The listing builds one solid part. Answer for the finished solid, in the listing's coordinates (mm). A direction names the side the tool comes from. Round coordinates to 2 decimals unless told otherwise and drop trailing zeros. Order: outer loops, then holes, each group sorted by start corner. A loop starts at its lowest first (then second) coordinate and runs counter-clockwise, first axis right, second up. Notation, with made-up numbers: (68.5, 34) - (100.5, 34) arc R10 cw to (100.5, 46) - close; hole circle Ø3 at (80.25, 35). An arc over 180 degrees is marked (long way). Use CSV: the item, a comma, the result in double quotes. Start each with the question number.
Item 1: Flat-ended cylindrical pins translate along their axes: P1, Ø8, axis at x = -41.5, y = 11, coming from the -Z side; P2, Ø7.5, axis at x = 50.8, z = 50.8, coming from the -Y side; P3, Ø13.5, axis at x = 41.275, z = -41.275, coming from the +Y side. Find the tip coordinate at first contact, or state that the pin passes through.
Item 2: Find section C-C, the plane z = 1. Give the vertices of the cut face in (x, y).
Item 3: For faces 4 (the cylindrical face through (-38.167, 3.335, 38.425)), 5 (the cylindrical face through (-51.35, -2.95, -54.98)), 6 (the cylindrical face through (-61.82, 0.14, -80.63)), determine the directions among +Z, -Z, +X, -X, +Y, -Y from which every point of the face is accessible in a straight line to the end or side of a thin tool.
Item 4: Straight lines are drawn through the part: line 1 along Z through (x, y) = (54, 0.5); line 2 along Z through (x, y) = (39.5, 5); line 3 along Y through (x, z) = (34, -81.5). For each, find the intervals that lie inside material, in ascending order. Write a range as [from, to].
Item 5: Determine the mould class of faces 1 (the conical face through (50.895, 6.157, 50.074)), 2 (the flat face through (76, 10.16, 15)), 3 (the cylindrical face through (46.367, 13.917, 60.47)) for opening direction X: +X half, -X half, draft (parallel to the pull), parting line (faces both ways), or undercut.
Item 6: Find section B-B, the plane y = 15.25. Give the vertices of the cut face in (x, z) (3 decimals).
Item 7: Find section A-A, the plane x = 0. Give the vertices of the cut face in (y, z) (3 decimals), plus the area to 3 significant figures.
Item 8: Find section D-D, the plane y = 0.25. Count the separate pieces of the cut face and the enclosed holes in it, plus the area to 3 significant figures.
```python
from build123d import *

# Parameters (mm, degrees)
SKETCH1_R                   = 101.6
BOSS_EXTRUDE1_DEPTH         = 10.16
F_3_8_24_TAPPED_HOLE2_D     = 8.4328
F_3_8_24_TAPPED_HOLE2_DEPTH = 13.462
F_3_8_24_TAPPED_HOLE2_TIP   = 2.533468714
F_3_8_24_TAPPED_HOLE1_D     = 8.4328
F_3_8_24_TAPPED_HOLE1_DEPTH = 14.224
F_3_8_24_TAPPED_HOLE1_TIP   = 2.533468714
SKETCH2_R                   = 76.2
SKETCH2_R_2                 = 73.025
BOSS_EXTRUDE2_DEPTH         = 7.62


with BuildPart() as part:
    # Sketch1 → Boss-Extrude1 (new, symmetric)
    with BuildSketch(Plane(origin=(0, 0, 0), x_dir=(1, 0, 0), z_dir=(0, 1, 0))):
        with Locations(Location((0, 0, 0), (0, 0, 270))):
            Circle(SKETCH1_R)
    extrude(amount=BOSS_EXTRUDE1_DEPTH, both=True)

    # 3/8-24 Tapped Hole2
    with Locations(Plane(origin=(0, 10.16, 0), x_dir=(1, 0, 0), z_dir=(0, 1, 0))):
        with Locations((-41.275, 41.275), (41.275, 41.275), (41.275, -41.275), (-41.275, -41.275)):
            Hole(F_3_8_24_TAPPED_HOLE2_D / 2, depth=F_3_8_24_TAPPED_HOLE2_DEPTH)
            with Locations((0, 0, -(F_3_8_24_TAPPED_HOLE2_DEPTH + F_3_8_24_TAPPED_HOLE2_TIP / 2))):  # 118° drill point
                Cone(0, F_3_8_24_TAPPED_HOLE2_D / 2, F_3_8_24_TAPPED_HOLE2_TIP, mode=Mode.SUBTRACT)

    # 3/8-24 Tapped Hole1
    with Locations(Plane(origin=(0, -10.16, 0), x_dir=(-1, 0, 0), z_dir=(0, -1, 0))):
        with Locations((50.8, -50.8), (-50.8, -50.8), (-50.8, 50.8), (50.8, 50.8)):
            Hole(F_3_8_24_TAPPED_HOLE1_D / 2, depth=F_3_8_24_TAPPED_HOLE1_DEPTH)
            with Locations((0, 0, -(F_3_8_24_TAPPED_HOLE1_DEPTH + F_3_8_24_TAPPED_HOLE1_TIP / 2))):  # 118° drill point
                Cone(0, F_3_8_24_TAPPED_HOLE1_D / 2, F_3_8_24_TAPPED_HOLE1_TIP, mode=Mode.SUBTRACT)

    # Sketch2 → Boss-Extrude2 (add)
    with BuildSketch(Plane(origin=(0, 10.16, 0), x_dir=(1, 0, 0), z_dir=(0, 1, 0))):
        with Locations(Location((0, 0, 0), (0, 0, 90))):
            Circle(SKETCH2_R)
        with Locations(Location((0, 0, 0), (0, 0, 90))):
            Circle(SKETCH2_R_2, mode=Mode.SUBTRACT)
    extrude(amount=BOSS_EXTRUDE2_DEPTH)


solid = part.part
```
Worked out:
1,P1,"stops at z = -94.39"
1,P2,"stops at y = 4.34"
1,P3,"stops at y = 10.16"
2,outline,"(-101.6, -10.16) - (101.6, -10.16) - (101.6, 10.16) - (76.19, 10.16) - (76.19, 17.78) - (73.02, 17.78) - (73.02, 10.16) - (-73.02, 10.16) - (-73.02, 17.78) - (-76.19, 17.78) - (-76.19, 10.16) - (-101.6, 10.16) - close"
3,face 4,"+Y"
3,face 5,"-Y"
3,face 6,"+Y, -Y"
4,line 1,"z = [-86.06, -53.55], [-48.05, 48.05], [53.55, 86.06]"
4,line 2,"z = [-93.61, -45.1], [-37.45, 37.45], [45.1, 93.61]"
4,line 3,"y = [-10.16, 10.16]"
5,face 1,"undercut"
5,face 2,"draft"
5,face 3,"parting line"
6,outline,"circle Ø152.4 at (0, 0); hole circle Ø146.05 at (0, 0)"
7,outline,"(-10.16, -101.6) - (10.16, -101.6) - (10.16, -76.2) - (17.78, -76.2) - (17.78, -73.025) - (10.16, -73.025) - (10.16, 73.025) - (17.78, 73.025) - (17.78, 76.2) - (10.16, 76.2) - (10.16, 101.6) - (-10.16, 101.6) - close"
7,area,"4,180 mm²"
8,separate pieces,"1"
8,enclosed holes,"8"
8,area,"32,000 mm²"
